from build123d import *

# Parameters (mm, degrees)
SKETCH1_R           = 29
BOSS_EXTRUDE1_DEPTH = 28
BOSS_EXTRUDE2_DEPTH = 52
SKETCH3_W           = 55
SKETCH3_H           = 55
BOSS_EXTRUDE3_DEPTH = 190
CIRPATTERN1_COUNT   = 6


with BuildPart() as part:
    # Sketch1 → Boss-Extrude1 (new body)
    with BuildSketch(Plane(origin=(0, 0, 0), x_dir=(1, 0, 0), z_dir=(0, 1, 0))):
        with Locations(Location((0, 0, 0), (0, 0, 270))):
            Circle(SKETCH1_R)
    extrude(amount=BOSS_EXTRUDE1_DEPTH)

    # Sketch2 → Boss-Extrude2 (add)
    with BuildSketch(Plane(origin=(0, 28, 0), x_dir=(1, 0, 0), z_dir=(0, 1, 0))):
        Polygon((24, 0), (24, 174), (-24, 174), (-24, 0), (-24, -217), (24, -217), align=None)
    boss_extrude2 = extrude(amount=BOSS_EXTRUDE2_DEPTH)

    # Sketch3 → Boss-Extrude3 (add)
    with BuildSketch(Plane(origin=(0, 80, 0), x_dir=(1, 0, 0), z_dir=(0, 1, 0))):
        with Locations((0, -145)):
            Rectangle(SKETCH3_W, SKETCH3_H)
    boss_extrude3 = extrude(amount=BOSS_EXTRUDE3_DEPTH)

    # CirPattern1: Boss-Extrude2, Boss-Extrude3 ×6 about axis
    cirpattern1_axis = Axis((0, 0, 0), (0, 1, 0))
    add([boss_extrude2.rotate(cirpattern1_axis, i * 360 / CIRPATTERN1_COUNT) for i in range(1, CIRPATTERN1_COUNT)])
    add([boss_extrude3.rotate(cirpattern1_axis, i * 360 / CIRPATTERN1_COUNT) for i in range(1, CIRPATTERN1_COUNT)])


solid = part.part
The listing builds one solid part. Answer for the finished solid, in the listing's coordinates (mm). A direction names the side the tool comes from. Give positions to 0.01 mm unless a question says otherwise; leave off trailing zeros. Write each loop counter-clockwise with the first axis right and the second up, starting at its lowest first coordinate (ties: lowest second). Pieces come first, ordered by that corner, then holes.
1) A tool of negligible diameter and unlimited length cuts with its end or side. For faces 1 (the face through (-1, 80, -195)), 2 (the face through (-98.9, 53.636, -84.813)), 3 (the face through (139.7, 173.7, 48.9)), 4 (the face through (168, 80, -97)), 5 (the face through (138, 80, -50)), from which of +Z, -Z, +X, -X, +Y, -Y can it reach the whole face along a straight path? Write none if from no direction.
2) Section D-D (z = 162) is taken. Write down the section's boundary in (x, y), and give its area (3 significant figures).
3) Section C-C (z = -47) is taken. Write down the section's boundary in (x, y).
4) Section B-B (x = 0) is taken. Write down the section's boundary in (y, z).
5) Section A-A (y = 176.5) is taken. Write down the section's boundary in (x, z), and give its area (4 significant figures).
6) Given P1, Ø10, axis at y = 27, z = -49.5, coming from the +X side; P2, Ø4, axis at x = 154.5, z = -69, coming from the -Y side; P3, Ø1.5, axis at y = 180.5, z = 33, coming from the +X side; P4, Ø1.5, axis at y = 145.5, z = 102.5, coming from the +X side, each flat-ended and moving along its own axis, determine where each tip first touches the part or whether it passes through.
7) Find the intervals of material crossed by L1, parallel to X at y = 37.5, z = 114.5; L2, parallel to Z at x = 8.5, y = 220.5; L3, parallel to X at y = 44, z = -93.5, in increasing order.
8) For a pull along Z with two mould halves and no side action, classify faces 6 (the face through (101.95, 173.67, -58.42)), 7 (the face through (-187.76, 53.64, -108.79)), 8 (the face through (-112, 80, 95)) as pulls with the +Z half, pulls with the -Z half, needs draft (parallel to the pull), parting line crosses it, or undercut.
Response:
1. face 1: -Z, +X, -X, +Y
1. face 2: -Z, -Y
1. face 3: +X, +Y, -Y
1. face 4: -Z, +X, +Y
1. face 5: +X, -Y
2. outline: (-27.5, 80) - (-24, 80) - (-24, 28) - (24, 28) - (24, 80) - (27.5, 80) - (27.5, 270) - (-27.5, 270) - close
2. area: 12,900 mm2
3. outline: (-136.41, 80) - (-129.41, 80) - (-129.41, 28) - (-33.41, 28) - (-33.41, 80) - (-108.54, 80) - (-108.54, 270) - (-136.41, 270) - close; (-24, 28) - (24, 28) - (24, 80) - (-24, 80) - close; (33.41, 28) - (129.41, 28) - (129.41, 80) - (136.41, 80) - (136.41, 270) - (108.54, 270) - (108.54, 80) - (33.41, 80) - close
4. outline: (0, -29) - (28, -29) - (28, -217) - (80, -217) - (80, -172.5) - (270, -172.5) - (270, -117.5) - (80, -117.5) - (80, 117.5) - (270, 117.5) - (270, 172.5) - (80, 172.5) - (80, 217) - (28, 217) - (28, 29) - (0, 29) - close
5. outline: (-163.14, -62.43) - (-135.64, -110.07) - (-88.01, -82.57) - (-115.51, -34.93) - close; (-163.14, 62.43) - (-115.51, 34.93) - (-88.01, 82.57) - (-135.64, 110.07) - close; (-27.5, -172.5) - (27.5, -172.5) - (27.5, -117.5) - (-27.5, -117.5) - close; (-27.5, 117.5) - (27.5, 117.5) - (27.5, 172.5) - (-27.5, 172.5) - close; (88.01, -82.57) - (135.64, -110.07) - (163.14, -62.43) - (115.51, -34.93) - close; (88.01, 82.57) - (115.51, 34.93) - (163.14, 62.43) - (135.64, 110.07) - close
5. area: 18,150 mm2
6. P1: stops at x = 142.22
6. P2: stops at y = 28
6. P3: passes through
6. P4: stops at x = 140.44
7. L1: x = -184.46 to -150.32, -24 to 24, 150.32 to 184.46
7. L2: z = -172.5 to -117.5, 117.5 to 172.5
7. L3: x = -196.59 to -113.95, -24 to 24, 113.95 to 196.59
8. face 6: undercut
8. face 7: pulls with the -Z half
8. face 8: needs draft
